The model under review builds one solid part; all positions refer to its coordinate system, in mm. Face numbers are marked on the shaded views. A direction names the side the tool comes from. Round coordinates to 2 decimals unless told otherwise and drop trailing zeros. Order: outer loops, then holes, each group sorted by start corner. A loop starts at its lowest first (then second) coordinate and runs counter-clockwise, first axis right, second up. Notation, with made-up numbers: M 60.5,45 L 64.5,45 A23 ccw 64.5,69 Z; hole C -20,22 d11. An arc over 180 degrees is marked long. Answer as a JSON object with one key per item and string values. Group by question number.
1) To check wall thickness, follow line 1 (Y direction, x = -21.5, z = 0.75); line 2 (Y direction, x = -17.5, z = 1.25); line 3 (Y direction, x = -9, z = 3). State the ranges of each line that lie inside material, in increasing order.
2) The part is to be moulded in two halves that separate along Y. For the marked faces 6, 7 and 8, say which applies: +Y half, -Y half, draft (parallel to the pull), parting line (faces both ways), or undercut.
3) For the marked faces 1, 2, 3, 4 and 5, list the 3-axis set-ups (+Z, -Z, +X, -X, +Y, -Y) from which the entire face can be reached by the end or side of a thin tool; tool diameter is ignored.
4) Consider section D-D, the plane x = 19. Write out the cut boundary in (y, z).
5) Consider section A-A, the plane z = 8.75. Write out the cut boundary in (x, y), then the cut area to 3 significant figures.
6) Insertion check: pin 1 Ø0.8 at (x, y) = (-18, -7.5) entering from +Z; pin 2 Ø0.9 at (y, z) = (6.5, 6.5) entering from +X; pin 3 Ø1.2 at (x, y) = (17.5, -6.5) entering from +Z. Each pin has a flat end and moves straight along its axis. Give the tip position at first contact, or say it passes through.
7) Consider section B-B, the plane x = 4. Write out the cut boundary in (y, z).
8) Consider section C-C, the plane y = -7. Write out the cut boundary in (x, z), then the cut area to 3 significant figures.
```python
from build123d import *

# Parameters (mm, degrees)
SKETCH1_W           = 45
SKETCH1_H           = 20
BOSS_EXTRUDE1_DEPTH = 1.5
SKETCH2_R           = 3
BOSS_EXTRUDE3_DEPTH = 8
SKETCH3_W           = 10
SKETCH3_H           = 3
BOSS_EXTRUDE4_DEPTH = 9
BOSS_EXTRUDE5_DEPTH = 6
SKETCH6_W           = 9
SKETCH6_H           = 7.5
BOSS_EXTRUDE6_DEPTH = 2.5
SKETCH7_W           = 1.5
SKETCH7_H           = 3
SKETCH7_W_2         = 3
SKETCH7_H_2         = 1.5
BOSS_EXTRUDE7_DEPTH = 1.5
SKETCH9_R           = 1.25
CUT_EXTRUDE1_DEPTH  = 0.5
SKETCH10_R          = 1.25
CUT_EXTRUDE2_DEPTH  = 0.5
SKETCH12_R          = 0.25
CUT_EXTRUDE3_DEPTH  = 1.5


with BuildPart() as part:
    # Sketch1 → Boss-Extrude1 (new body)
    with BuildSketch(Plane.XY):
        Rectangle(SKETCH1_W, SKETCH1_H)
    extrude(amount=BOSS_EXTRUDE1_DEPTH)

    # Sketch2 → Boss-Extrude3 (add)
    with BuildSketch(Plane.XY.offset(1.5)):
        with Locations((-18.5, 0)):
            Circle(SKETCH2_R)
        with Locations(Location((18.5, 0, 0), (0, 0, 180))):
            Circle(SKETCH2_R)
    extrude(amount=BOSS_EXTRUDE3_DEPTH)

    # Sketch3 → Boss-Extrude4 (add)
    with BuildSketch(Plane.XY.offset(1.5)):
        with Locations((-8.5, 6)):
            Rectangle(SKETCH3_W, SKETCH3_H)
    extrude(amount=BOSS_EXTRUDE4_DEPTH)

    # Sketch5 → Boss-Extrude5 (add)
    with BuildSketch(Plane.XY.offset(1.5)):
        with BuildLine():
            Line((-12, 1), (-4, 1))
            ThreePointArc((-4, 1), (-2.585786438, 0.414213562), (-2, -1))
            Line((-2, -1), (-2, -6))
            ThreePointArc((-2, -6), (-2.585786438, -7.414213562), (-4, -8))
            Line((-4, -8), (-12, -8))
            ThreePointArc((-12, -8), (-13.414213562, -7.414213562), (-14, -6))
            Line((-14, -6), (-14, -1))
            ThreePointArc((-14, -1), (-13.414213562, 0.414213562), (-12, 1))
        make_face()
    extrude(amount=BOSS_EXTRUDE5_DEPTH)

    # Sketch6 → Boss-Extrude6 (add)
    with BuildSketch(Plane.XY.offset(1.5)):
        with Locations((7, 3.75)):
            Rectangle(SKETCH6_W, SKETCH6_H)
    extrude(amount=BOSS_EXTRUDE6_DEPTH)

    # Sketch7 → Boss-Extrude7 (add)
    with BuildSketch(Plane.XY.offset(1.5)):
        with Locations((17.75, -6.5)):
            Rectangle(SKETCH7_W, SKETCH7_H)
        with Locations((10, -5.25)):
            Rectangle(SKETCH7_W_2, SKETCH7_H_2)
    extrude(amount=BOSS_EXTRUDE7_DEPTH)

    # Sketch9 → Cut-Extrude1 (cut)
    with BuildSketch(Plane.XY.offset(1.5)):
        with Locations((-17.5, -7)):
            Circle(SKETCH9_R)
    extrude(amount=-CUT_EXTRUDE1_DEPTH, mode=Mode.SUBTRACT)

    # Sketch10 → Cut-Extrude2 (cut)
    with BuildSketch(Plane.XY.offset(1.5)):
        with Locations((16, 6.5)):
            Circle(SKETCH10_R)
    extrude(amount=-CUT_EXTRUDE2_DEPTH, mode=Mode.SUBTRACT)

    # Sketch12 → Cut-Extrude3 (cut)
    with BuildSketch(Plane.XY.offset(1.5)):
        with Locations((-21.5, 9)):
            Circle(SKETCH12_R)
        with Locations((21.5, 9)):
            Circle(SKETCH12_R)
        with Locations((21.5, -9)):
            Circle(SKETCH12_R)
        with Locations((-21.5, -9)):
            Circle(SKETCH12_R)
    extrude(amount=-CUT_EXTRUDE3_DEPTH, mode=Mode.SUBTRACT)


solid = part.part
```
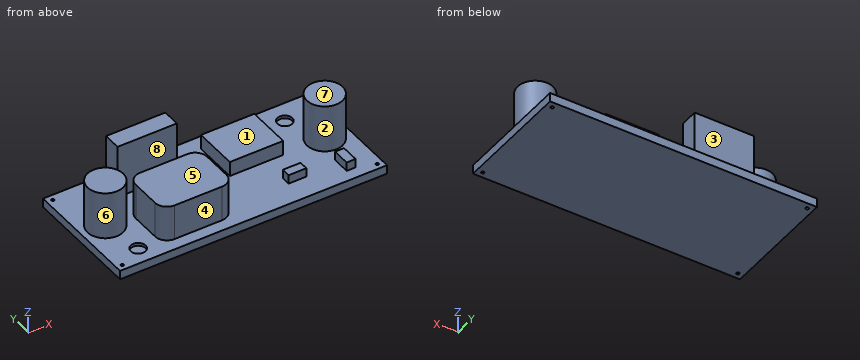
Results list:
{
 "1": {"line 1": "-10 to -9.25, -8.75 to 8.75, 9.25 to 10", "line 2": "-10 to -8.25, -5.75 to 10", "line 3": "-8 to 1, 4.5 to 7.5"},
 "2": {"face 6": "parting line", "face 7": "draft", "face 8": "undercut"},
 "3": {"face 1": "+Z, +Y, -Y", "face 2": "+Z", "face 3": "+Z, +X, -X, +Y", "face 4": "+Z, +X, -X, -Y", "face 5": "+Z, -Y"},
 "4": {"outline": "M -10,0 L 10,0 L 10,1.5 L 2.96,1.5 L 2.96,9.5 L -2.96,9.5 L -2.96,1.5 L -10,1.5 Z"},
 "5": {"outline": "C -18.5,0 d6; M -13.5,4.5 L -3.5,4.5 L -3.5,7.5 L -13.5,7.5 Z; C 18.5,0 d6", "area": "86.5 mm^2"},
 "6": {"pin 1": "z = 1", "pin 2": "x = -3.5", "pin 3": "z = 3"},
 "7": {"outline": "M -10,0 L 10,0 L 10,1.5 L 7.5,1.5 L 7.5,4 L 0,4 L 0,1.5 L -10,1.5 Z"},
 "8": {"outline": "M -22.5,0 L 22.5,0 L 22.5,1.5 L 18.5,1.5 L 18.5,3 L 17,3 L 17,1.5 L -2.27,1.5 L -2.27,7.5 L -13.73,7.5 L -13.73,1.5 L -16.25,1.5 L -16.25,1 L -18.75,1 L -18.75,1.5 L -22.5,1.5 Z", "area": "137 mm^2"}
}
